```python
from build123d import *

# Parameters (mm, degrees)
SKETCH1_R           = 15
BOSS_EXTRUDE1_DEPTH = 0.9652
SKETCH2_R           = 1.6
BOSS_EXTRUDE2_DEPTH = 0.9652
SKETCH3_W           = 30
SKETCH3_H           = 26
BOSS_EXTRUDE3_DEPTH = 0.9652
SKETCH4_R           = 14.6
BOSS_EXTRUDE4_DEPTH = 16.0348
SKETCH5_R           = 1.5
BOSS_EXTRUDE5_DEPTH = 11
SKETCH6_R           = 7
BOSS_EXTRUDE6_DEPTH = 2
BOSS_EXTRUDE7_DEPTH = 4.445


with BuildPart() as part:
    # Sketch1 → Boss-Extrude1 (new body)
    with BuildSketch(Plane.XY):
        with Locations(Location((0, 0, 0), (0, 0, 180))):
            Circle(SKETCH1_R)
    extrude(amount=BOSS_EXTRUDE1_DEPTH)

    # Sketch2 → Boss-Extrude2 (add, through all)
    with BuildSketch(Plane.XY.offset(0.9652)):
        with BuildLine():
            Line((-21.315789474, 3.26145966), (-8.684210526, 12.230473725))
            ThreePointArc((-8.684210526, 12.230473725), (0, 15), (8.684210526, 12.230473725))
            Line((8.684210526, 12.230473725), (21.315789474, 3.26145966))
            ThreePointArc((21.315789474, 3.26145966), (23, 0), (21.315789474, -3.26145966))
            Line((21.315789474, -3.26145966), (8.684210526, -12.230473725))
            ThreePointArc((8.684210526, -12.230473725), (0, -15), (-8.684210526, -12.230473725))
            Line((-8.684210526, -12.230473725), (-21.315789474, -3.26145966))
            ThreePointArc((-21.315789474, -3.26145966), (-23, 0), (-21.315789474, 3.26145966))
        make_face()
        with Locations((-19, 0)):
            Circle(SKETCH2_R, mode=Mode.SUBTRACT)
        with Locations((19, 0)):
            Circle(SKETCH2_R, mode=Mode.SUBTRACT)
    extrude(amount=-BOSS_EXTRUDE2_DEPTH)

    # Sketch3 → Boss-Extrude3 (add, through all)
    with BuildSketch(Plane.XY.offset(0.9652)):
        with Locations((0, -15)):
            Rectangle(SKETCH3_W, SKETCH3_H)
    extrude(amount=-BOSS_EXTRUDE3_DEPTH)

    # Sketch4 → Boss-Extrude4 (add)
    with BuildSketch(Plane.XY.offset(0.9652)):
        Circle(SKETCH4_R)
    extrude(amount=BOSS_EXTRUDE4_DEPTH)

    # Sketch5 → Boss-Extrude5 (add)
    with BuildSketch(Plane(origin=(0, 0, 0), x_dir=(-1, 0, 0), z_dir=(0, 0, -1))):
        with Locations(Location((0, 0, 0), (0, 0, 180))):
            Circle(SKETCH5_R)
    extrude(amount=BOSS_EXTRUDE5_DEPTH)

    # Sketch6 → Boss-Extrude6 (add)
    with BuildSketch(Plane(origin=(0, 0, 0), x_dir=(-1, 0, 0), z_dir=(0, 0, -1))):
        with Locations(Location((0, 0, 0), (0, 0, 180))):
            Circle(SKETCH6_R)
    extrude(amount=BOSS_EXTRUDE6_DEPTH)

    # Sketch7 → Boss-Extrude7 (add, symmetric)
    with BuildSketch(Plane(origin=(0, 0, 0), x_dir=(0, 0, -1), z_dir=(1, 0, 0))):
        with BuildLine():
            Line((-48.879875, -11.826), (-39.989875, -11.826))
            ThreePointArc((-39.989875, -11.826), (-30.420049501, -14.417177809), (-23.46493471, -21.482737995))
            Line((-23.46493471, -21.482737995), (-22.44314029, -23.296262005))
            ThreePointArc((-22.44314029, -23.296262005), (-15.488025499, -30.361822191), (-5.9182, -32.953))
            ThreePointArc((-5.9182, -32.953), (-2.415900113, -31.502299887), (-0.9652, -28))
            Line((-0.9652, -28), (-0.9652, -17.872983346))
            Line((-0.9652, -17.872983346), (-1.0922, -17.872983346))
            Line((-1.0922, -17.872983346), (-1.0922, -28))
            ThreePointArc((-1.0922, -28), (-2.505702674, -31.412497326), (-5.9182, -32.826))
            ThreePointArc((-5.9182, -32.826), (-15.423948796, -30.252171946), (-22.332494209, -23.233920647))
            Line((-22.332494209, -23.233920647), (-23.35428863, -21.420396638))
            ThreePointArc((-23.35428863, -21.420396638), (-30.355972799, -14.307527564), (-39.989875, -11.699))
            Line((-39.989875, -11.699), (-48.879875, -11.699))
            Line((-48.879875, -11.699), (-48.879875, -11.826))
        make_face()
    extrude(amount=BOSS_EXTRUDE7_DEPTH, both=True)


solid = part.part
```
The model under review builds one solid part; all positions refer to its coordinate system, in mm. A direction names the side the tool comes from. Round coordinates to 2 decimals unless told otherwise and drop trailing zeros. Loops run counter-clockwise (first coordinate to the right, second up) from the corner with the lowest first, then second, coordinate; pieces in that order, holes last. Notation, with made-up numbers: (55.5, 19) -> (63.5, 19) arc R25 ccw to (63.5, 48) -> close; hole circle Ø10 at (81, -17). An arc over 180 degrees is marked (long way). Answer in a Markdown table with one row per item.
1) Draft analysis for pull direction X (two halves, no side actions). For faces 1 (the flat face through (18.202, -5.472, 0.489)), 2 (the cylindrical face through (-23, -0.1, 0.5)), 3 (the cylindrical face through (-20.18, 1.08, 0.49)), state which applies: pulls with the +X half, pulls with the -X half, needs draft (parallel to the pull), parting line crosses it, or undercut.
Taken from the geometry:
| item | result |
|---|---|
| face 1 | pulls with the +X half |
| face 2 | pulls with the -X half |
| face 3 | undercut |
2) Wall thickness on line 1 along Z through (x, y) = (2, 5.5); line 2 along Z through (x, y) = (-9, -17); line 3 along Y through (x, z) = (19, 0.55): over which ranges is each line inside the solid? List them lowest first.
Taken from the geometry:
| item | result |
|---|---|
| line 1 | z = -2 to 17 |
| line 2 | z = 0 to 0.97 |
| line 3 | y = -4.91 to -1.6, 1.6 to 4.91 |
3) For pin 1 Ø6 at (y, z) = (-8, 18.5) entering from +X; pin 2 Ø6.5 at (y, z) = (-21, 23.5) entering from +X (3 decimals); pin 3 Ø2 at (x, y) = (13.5, -22.5) entering from +Z, all flat-tipped, find the tip position at first contact; note any pin that passes through.
Taken from the geometry:
| item | result |
|---|---|
| pin 1 | stops at x = 13.56 |
| pin 2 | stops at x = 4.445 |
| pin 3 | stops at z = 0.97 |
4) Consider section D-D, the plane z = 31. Write out the cut boundary in (x, y) (3 decimals).
Taken from the geometry:
| item | result |
|---|---|
| outline | (-4.445, -14.092) -> (4.445, -14.092) -> (4.445, -13.948) -> (-4.445, -13.948) -> close |
5) Consider section B-B, the plane x = 19.5. Write out the cut boundary in (y, z), plus the area to 3 significant figures.
Taken from the geometry:
| item | result |
|---|---|
| outline | (-4.55, 0) -> (-1.52, 0) -> (-1.52, 0.97) -> (-4.55, 0.97) -> close; (1.52, 0) -> (4.55, 0) -> (4.55, 0.97) -> (1.52, 0.97) -> close |
| area | 5.85 mm² |
6) Tool access review of faces 4 (the cylindrical face through (1.43, -0.45, -6.44)), 5 (the flat face through (14.91, 7.81, 0.49)): name each direction out of +Z, -Z, +X, -X, +Y, -Y from which nothing blocks a thin tool from reaching the whole face with its end or side.
Taken from the geometry:
| item | result |
|---|---|
| face 4 | -Z |
| face 5 | +Z, -Z, +X, +Y |
7) Consider section A-A, the plane y = 0. Write out the cut boundary in (x, z), plus the area to 3 significant figures.
Taken from the geometry:
| item | result |
|---|---|
| outline | (-23, 0) -> (-20.6, 0) -> (-20.6, 0.97) -> (-23, 0.97) -> close; (-17.4, 0) -> (-7, 0) -> (-7, -2) -> (-1.5, -2) -> (-1.5, -11) -> (1.5, -11) -> (1.5, -2) -> (7, -2) -> (7, 0) -> (17.4, 0) -> (17.4, 0.97) -> (14.6, 0.97) -> (14.6, 17) -> (-14.6, 17) -> (-14.6, 0.97) -> (-17.4, 0.97) -> close; (20.6, 0) -> (23, 0) -> (23, 0.97) -> (20.6, 0.97) -> close |
| area | 561 mm² |
